For this review, take the finished solid that the model builds, in its own axes (mm). A direction names the side the tool comes from. Coordinates: 2 decimals unless noted, no trailing zeros. Loops run counter-clockwise (first coordinate to the right, second up) from the corner with the lowest first, then second, coordinate; pieces in that order, holes last. Notation, with made-up numbers: (-35.75, 54.5) -> (-21.75, 54.5) arc R19 ccw to (-21.75, 78.5) -> close; hole circle Ø6 at (80, 19). An arc over 180 degrees is marked (long way). Answer in a Markdown table with one row per item.
from build123d import *

# Parameters (mm, degrees)
F0_W     = 76
F0_H     = 156
F1_DEPTH = 2.5
F0_W_2   = 80
F0_H_2   = 160
F2_DEPTH = 35
F4_DEPTH = 160


with BuildPart() as f1:
    # F0 (on Top) → F1 (new body)
    with BuildSketch(Plane.XY):
        with Locations((-62.088289, -6.299588)):
            Rectangle(F0_W, F0_H)
    extrude(amount=F1_DEPTH)

    # F0 (on Top) → F2 (join)
    with BuildSketch(Plane.XY):
        with Locations((-62.088289, -6.299588)):
            Rectangle(F0_W_2, F0_H_2)
        with Locations((-62.088289, -6.299588)):
            Rectangle(F0_W, F0_H, mode=Mode.SUBTRACT)
    extrude(amount=F2_DEPTH)

    # F3 (on face) → F4 (cut)
    with BuildSketch(Plane.XZ.offset(86.299588)):
        with BuildLine():
            ThreePointArc((-80.088289, 35), (-62.088289, 17), (-44.088289, 35))
            Line((-44.088289, 35), (-80.088289, 35))
        make_face()
    extrude(amount=-F4_DEPTH, mode=Mode.SUBTRACT)


solid = f1.part
Item 1: Insertion check: pin 1 (5 mm diameter, centred on x = -43.5, y = -44, fed in from +Z). The pin has a flat end and moves straight along its axis. Give the tip position at first contact, or say it passes through.
Worked answers:
| item | result |
|---|---|
| pin 1 | z = 2.5 |
Item 2: Take a section at A-A, the plane z = 11.5. State the section outline as (x, y) points, and give its area (3 significant figures).
Worked answers:
| item | result |
|---|---|
| outline | (-102.09, -86.3) -> (-22.09, -86.3) -> (-22.09, 73.7) -> (-102.09, 73.7) -> close; hole (-100.09, -84.3) -> (-24.09, -84.3) -> (-24.09, 71.7) -> (-100.09, 71.7) -> close |
| area | 944 mm² |
Item 3: Take a section at C-C, the plane z = 31.5. State the section outline as (x, y) points.
Worked answers:
| item | result |
|---|---|
| outline | (-102.09, -86.3) -> (-79.74, -86.3) -> (-79.74, -84.3) -> (-100.09, -84.3) -> (-100.09, 71.7) -> (-79.74, 71.7) -> (-79.74, 73.7) -> (-102.09, 73.7) -> close; (-44.43, -86.3) -> (-22.09, -86.3) -> (-22.09, 73.7) -> (-44.43, 73.7) -> (-44.43, 71.7) -> (-24.09, 71.7) -> (-24.09, -84.3) -> (-44.43, -84.3) -> close |
Item 4: The part is to be moulded in two halves that separate along X. For faces 3 (the flat face through (-102.088, -7, 17)), 4 (the flat face through (-23, -6, 35)), 5 (the flat face through (-63, -84.3, 15)), say which applies: +X half, -X half, draft (parallel to the pull), parting line (faces both ways), or undercut.
Worked answers:
| item | result |
|---|---|
| face 3 | -X half |
| face 4 | draft |
| face 5 | undercut |
Item 5: Take a section at B-B, the plane y = -74. State the section outline as (x, z) points, and give its area (3 significant figures).
Worked answers:
| item | result |
|---|---|
| outline | (-102.09, 0) -> (-22.09, 0) -> (-22.09, 35) -> (-24.09, 35) -> (-24.09, 2.5) -> (-100.09, 2.5) -> (-100.09, 35) -> (-102.09, 35) -> close |
| area | 330 mm² |
Item 6: Take a section at D-D, the plane x = -92.5. State the section outline as (y, z) points.
Worked answers:
| item | result |
|---|---|
| outline | (-86.3, 0) -> (73.7, 0) -> (73.7, 35) -> (71.7, 35) -> (71.7, 2.5) -> (-84.3, 2.5) -> (-84.3, 35) -> (-86.3, 35) -> close |
Item 7: For faces 1 (the flat face through (-63, -5, 2.5)), 2 (the cylindrical face through (-62, -85, 17)), list the 3-axis set-ups (+Z, -Z, +X, -X, +Y, -Y) from which the entire face can be reached by the end or side of a thin tool; tool diameter is ignored.
Worked answers:
| item | result |
|---|---|
| face 1 | +Z |
| face 2 | +Z, +Y, -Y |
Item 8: For L1, parallel to X at y = 10, z = 8.5; L2, parallel to Y at x = -60.5, z = 7.5; L3, parallel to Z at x = -57, y = -14.5, list the stretches that pass through material, from the lowest coordinate up.
Worked answers:
| item | result |
|---|---|
| L1 | -102.09 to -100.09, -24.09 to -22.09 |
| L2 | -86.3 to -84.3, 71.7 to 73.7 |
| L3 | 0 to 2.5 |
